Design review of the part built by this model. Coordinates are the model's own, in mm. Face numbers are marked on the shaded views. A direction names the side the tool comes from. Give positions to 0.01 mm unless a question says otherwise; leave off trailing zeros. Order: outer loops, then holes, each group sorted by start corner. A loop starts at its lowest first (then second) coordinate and runs counter-clockwise, first axis right, second up. Notation, with made-up numbers: M -8,65 L 6,65 A18 cw 6,78 Z; hole C 44,-11.5 d3. An arc over 180 degrees is marked long. Put each result on its own line as item: value. Start each with the question number.
from build123d import *

# Parameters (mm, degrees)
F0_R     = 9
F0_R_2   = 7.75
F1_DEPTH = 2.5
F3_DEPTH = 25
F4_W     = 1.797143
F4_H     = 0.470712
F5_DEPTH = 25
F6_W     = 1.035781
F6_H     = 1.391272
F7_DEPTH = 25


with BuildPart() as f1:
    # F0 (on Front) → F1 (new body)
    with BuildSketch(Plane.XZ):
        Circle(F0_R)
        Circle(F0_R_2, mode=Mode.SUBTRACT)
    extrude(amount=F1_DEPTH)

    # F2 (on face) → F3 (cut)
    with BuildSketch(Plane.XZ.offset(2.5)):
        Polygon((-6.525024, 6.198715), (-7.695748, 4.666418), (-6.611456, 4.043655), (-5.404168, 5.55495), align=None)
    extrude(amount=-F3_DEPTH, mode=Mode.SUBTRACT)

    # F4 (on face) → F5 (cut)
    with BuildSketch(Plane.XZ.offset(2.5)):
        with Locations((-7.423595, 5.963359)):
            Rectangle(F4_W, F4_H)
    extrude(amount=-F5_DEPTH, mode=Mode.SUBTRACT)

    # F6 (on face) → F7 (cut)
    with BuildSketch(Plane.XZ.offset(2.5)):
        with Locations((-7.177858, 5.362054)):
            Rectangle(F6_W, F6_H)
    extrude(amount=-F7_DEPTH, mode=Mode.SUBTRACT)


solid = f1.part
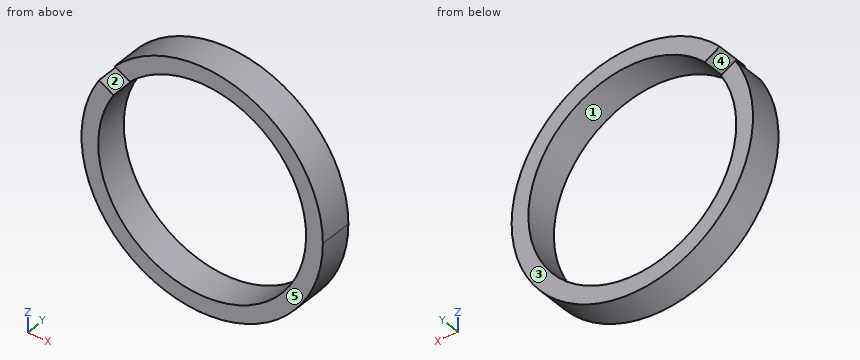
1. Consider section C-C on y = -2.15. Give the boundary of the cut face in (x, z), then the cut area to 3 significant figures.
2. Consider section A-A on x = 0. Give the boundary of the cut face in (y, z), then the cut area to 3 significant figures.
3. The part is to be moulded in two halves that separate along Z. For the marked faces 1, 2 and 3, say which applies: +Z half, -Z half, draft (parallel to the pull), parting line (faces both ways), or undercut.
4. To check wall thickness, follow probe 1 along X at (y, z) = (-0.6, 0); probe 2 along X at (y, z) = (-1.45, -2). State the ranges of each line that lie inside material, in increasing order.
5. Machinability: for the marked faces 4 and 5, which of the approach directions +Z, -Z, +X, -X, +Y, -Y give a long, thin tool a straight path to every point of the face, cutting with its end or side? Answer none if there is none.
6. Consider section B-B on z = 6.5. Give the boundary of the cut face in (x, y).
Returned:
1. outline: M -7.7,4.67 A9 ccw long -6.53,6.2 L -5.4,5.55 A7.75 cw long -6.61,4.04 Z
1. area: 63.4 mm2
2. outline: M -2.5,-9 L 0,-9 L 0,-7.75 L -2.5,-7.75 Z; M -2.5,7.75 L 0,7.75 L 0,9 L -2.5,9 Z
2. area: 6.25 mm2
3. face 1: undercut
3. face 2: +Z half
3. face 3: draft
4. probe 1: x = -9 to -7.75, 7.75 to 9
4. probe 2: x = -8.77 to -7.49, 7.49 to 8.77
5. face 4: -X, +Y, -Y
5. face 5: +Z, -Z, +X, -X, -Y
6. outline: M -6.22,-2.5 L -4.22,-2.5 L -4.22,0 L -6.22,0 Z; M 4.22,-2.5 L 6.22,-2.5 L 6.22,0 L 4.22,0 Z
